Could you check a few things on this model? Use its own coordinates, in mm. Give positions to 0.01 mm unless a question says otherwise; leave off trailing zeros. Order: outer loops, then holes, each group sorted by start corner. A loop starts at its lowest first (then second) coordinate and runs counter-clockwise, first axis right, second up. Notation, with made-up numbers: M 54,45.5 L 108,45.5 A31 ccw 108,77.5 Z; hole C 1,31.25 d10. An arc over 180 degrees is marked long. Answer in a Markdown table with one row per item. Add a question column.
```python
from build123d import *

# Parameters (mm, degrees)
BASPROSKE_W         = 4
BASPROSKE_H         = 10.5
TOOTHCUT_DEPTH      = 16.378556499
TEETHCUTS_COUNT     = 10
TEETHCUTS_ANGLE     = 324
BORSKE_R            = 0.5
BORE_DEPTH          = 50.0000508
BOSS_EXTRUDE1_START = -4.3
SKETCH2_R           = 0.5
BOSS_EXTRUDE1_DEPTH = 4.3
SKETCH2_3_R         = 0.5
BOSS_EXTRUDE2_DEPTH = 9.9


with BuildPart() as part:
    # BasProSke → Base-Revolve (revolve)
    with BuildSketch(Plane(origin=(0, 0, 0), x_dir=(1, 0, 0), z_dir=(0, 1, 0)), mode=Mode.PRIVATE) as base_revolve_sk:
        with Locations((2, 5.25)):
            Rectangle(BASPROSKE_W, BASPROSKE_H)
    revolve(base_revolve_sk.sketch.rotate(Axis((-10, 0, 0), (1, 0, 0)), 180), axis=Axis((-10, 0, 0), (1, 0, 0)))

    # TooCutSke → ToothCut (cut, through all)
    with BuildSketch(Plane(origin=(0, 0, 0), x_dir=(0, 0, -1), z_dir=(1, 0, 0))):
        with BuildLine():
            ThreePointArc((1.019600066, 6.481797432), (0, 6.5615), (-1.019600066, 6.481797432))
            ThreePointArc((-1.019600066, 6.481797432), (-1.451036104, 8.608938557), (-3.053606956, 10.072712133))
            ThreePointArc((-3.053606956, 10.072712133), (0, 10.5254), (3.053606956, 10.072712133))
            ThreePointArc((3.053606956, 10.072712133), (1.451036104, 8.608938557), (1.019600066, 6.481797432))
        make_face()
    toothcut = extrude(amount=TOOTHCUT_DEPTH, mode=Mode.SUBTRACT)

    # TeethCuts: ToothCut ×10 about axis
    teethcuts_axis = Axis((-10, 0, 0), (1, 0, 0))
    for i in range(1, TEETHCUTS_COUNT):
        add(toothcut.rotate(teethcuts_axis, i * TEETHCUTS_ANGLE / (TEETHCUTS_COUNT - 1)), mode=Mode.SUBTRACT)

    # BorSke → Bore (cut, symmetric)
    with BuildSketch(Plane(origin=(0, 0, 0), x_dir=(0, 0, -1), z_dir=(1, 0, 0))):
        with Locations(Location((0, 0, 0), (0, 0, 180))):
            Circle(BORSKE_R)
    extrude(amount=BORE_DEPTH, both=True, mode=Mode.SUBTRACT)

    # Sketch2 → Boss-Extrude1 (add)
    # profile 1 of 8: a face of its own
    with BuildSketch(Plane.ZY.offset(BOSS_EXTRUDE1_START)):
        with BuildLine():
            ThreePointArc((-0.75, -0.433012702), (-0.433012702, -0.75), (0, -0.866025404))
            Line((0, -0.866025404), (-0.75, -0.433012702))
        make_face()
    # profile 2 of 8: a face of its own
    with BuildSketch(Plane.ZY.offset(BOSS_EXTRUDE1_START)):
        Polygon((0, -0.866025404), (0.75, -0.433012702), (0.75, 0.433012702), (0, 0.866025404), (-0.75, 0.433012702), (-0.75, -0.433012702), align=None)
        Circle(SKETCH2_R, mode=Mode.SUBTRACT)
    # profile 3 of 8: a face of its own
    with BuildSketch(Plane.ZY.offset(BOSS_EXTRUDE1_START)):
        with BuildLine():
            Line((-0.75, -0.433012702), (-0.75, 0.433012702))
            ThreePointArc((-0.75, 0.433012702), (-0.866025404, 0), (-0.75, -0.433012702))
        make_face()
    # profile 4 of 8: a face of its own
    with BuildSketch(Plane.ZY.offset(BOSS_EXTRUDE1_START)):
        with BuildLine():
            Line((-0.75, 0.433012702), (0, 0.866025404))
            ThreePointArc((0, 0.866025404), (-0.433012702, 0.75), (-0.75, 0.433012702))
        make_face()
    # profile 5 of 8: a face of its own
    with BuildSketch(Plane.ZY.offset(BOSS_EXTRUDE1_START)):
        with BuildLine():
            Line((0, 0.866025404), (0.75, 0.433012702))
            ThreePointArc((0.75, 0.433012702), (0.433012702, 0.75), (0, 0.866025404))
        make_face()
    # profile 6 of 8: a face of its own
    with BuildSketch(Plane.ZY.offset(BOSS_EXTRUDE1_START)):
        with BuildLine():
            ThreePointArc((0.866025404, 0), (0.836516304, 0.224143868), (0.75, 0.433012702))
            Line((0.75, 0.433012702), (0.75, -0.433012702))
            ThreePointArc((0.75, -0.433012702), (0.836516304, -0.224143868), (0.866025404, 0))
        make_face()
    # profile 7 of 8: a face of its own
    with BuildSketch(Plane.ZY.offset(BOSS_EXTRUDE1_START)):
        with BuildLine():
            ThreePointArc((0, -0.866025404), (0.433012702, -0.75), (0.75, -0.433012702))
            Line((0.75, -0.433012702), (0, -0.866025404))
        make_face()
    # profile 8 of 8: a face of its own
    with BuildSketch(Plane.ZY.offset(BOSS_EXTRUDE1_START)):
        Circle(SKETCH2_R)
    extrude(amount=BOSS_EXTRUDE1_DEPTH)

    # Sketch2_3 → Boss-Extrude2 (add)
    # profile 1 of 2: a face of its own
    with BuildSketch(Plane.ZY):
        Polygon((0, -0.866025404), (0.75, -0.433012702), (0.75, 0.433012702), (0, 0.866025404), (-0.75, 0.433012702), (-0.75, -0.433012702), align=None)
        Circle(SKETCH2_3_R, mode=Mode.SUBTRACT)
    # profile 2 of 2: a face of its own
    with BuildSketch(Plane.ZY):
        Circle(SKETCH2_3_R)
    extrude(amount=-BOSS_EXTRUDE2_DEPTH)


solid = part.part
```
1. Thinking about a two-plate mould opening in Z: for faces 1 (the flat face through (4, -2, 0)), 2 (the flat face through (7, 0, 0.75)), 3 (the cylindrical face through (1.97, -6.56, 0.01)), which applies, pulls with the +Z half, pulls with the -Z half, needs draft (parallel to the pull), parting line crosses it, or undercut?
2. Suppose I cut it at A-A on x = 8.75. List the corners of the cut face in (y, z) for me, plus the area to 3 significant figures.
3. If I drill on line 1 along Z through (x, y) = (1.75, 6); line 2 along X through (y, z) = (0.5, -5.5); line 3 along Y through (x, z) = (1, 3.5), over which ranges is the centre line in solid material (lowest first)? Write a range as [from, to].
4. Suppose I cut it at C-C on z = -5.25. List the corners of the cut face in (x, y) for me.
5. Suppose I cut it at B-B on y = 8.5. List the corners of the cut face in (x, z) for me, plus the area to 3 significant figures.
6. Will these pins go through, and if not, where does the flat tip stop? P1, Ø1, axis at x = 2.5, y = -5, coming from the +Z side; P2, Ø4, axis at x = 8, z = -2.5, coming from the +Y side; P3, Ø1, axis at x = 8, y = 0, coming from the +Z side.
7. Suppose I cut it at D-D on y = 4. List the corners of the cut face in (x, z) for me.
Findings below:
| question | item | result |
|---|---|---|
| 1 | face 1 | needs draft |
| 1 | face 2 | pulls with the +Z half |
| 1 | face 3 | undercut |
| 2 | outline | M -0.87,0 L -0.43,-0.75 L 0.43,-0.75 L 0.87,0 L 0.43,0.75 L -0.43,0.75 Z |
| 2 | area | 1.95 mm2 |
| 3 | line 1 | [-8.62, -6.01], [-3.12, 3.12], [6.01, 8.62] |
| 3 | line 2 | [0, 4] |
| 3 | line 3 | [-9.85, -6.57], [-5.55, 5.55], [6.57, 9.85] |
| 4 | outline | M 0,-5.44 L 4,-5.44 L 4,5.44 L 0,5.44 Z |
| 5 | outline | M 0,-3.9 L 4,-3.9 L 4,-1.39 L 0,-1.39 Z; M 0,1.39 L 4,1.39 L 4,3.9 L 0,3.9 Z |
| 5 | area | 20.0 mm2 |
| 6 | P1 | z = 8.54 |
| 6 | P2 | y = 0.58 |
| 6 | P3 | z = 0.75 |
| 7 | outline | M 0,-7.7 L 4,-7.7 L 4,7.7 L 0,7.7 Z |
